Here's how the part is built. I have some questions about the finished solid (model axes, mm). Give positions to 0.01 mm unless a question says otherwise; leave off trailing zeros. Loops run counter-clockwise (first coordinate to the right, second up) from the corner with the lowest first, then second, coordinate; pieces in that order, holes last. Notation, with made-up numbers: (-39, 25) -> (-9, 25) arc R28 cw to (-9, 48) -> close; hole circle Ø10 at (88.5, -4). An arc over 180 degrees is marked (long way). Answer in a Markdown table with one row per item. Add a question column.
Item 1: If we section it at C-C (z = 13): Write out the boundary of the cut face in (x, y), then the cut area to 3 significant figures.
Item 2: If we section it at D-D (y = 132.5): Write out the boundary of the cut face in (x, z), then the cut area to 3 significant figures.
Item 3: If we section it at B-B (x = 10): Give the number of separate pieces and of enclosed holes in the cut face, then the cut area to 3 significant figures.
Item 4: If I drill on line 1 (Y direction, x = 6, z = 18); line 2 (Z direction, x = 1.75, y = 152); line 3 (Z direction, x = 7.25, y = 154), over which ranges is the centre line in solid material (lowest first)?
Item 5: If we section it at A-A (z = 18.75): Write out the boundary of the cut face in (x, y).
Item 6: We'd pull the mould along Y, two halves only. Please class faces 1 (the face through (10.14, 152.857, 4.608)), 2 (the face through (10, 151, 30)), 3 (the face through (10, 176.376, 14)), 4 (the face through (10.14, 127.33, 29.095)): released by +Y, released by -Y, zero draft, split by the parting line, or undercut.
Autodesk Inventor part; units mm, degrees
ref_plane "YZ Plane" through (0, 0, 0) normal (1, 0, 0) x (0, 1, 0)
ref_plane "XZ Plane" through (0, 0, 0) normal (0, 1, 0) x (-1, 0, 0)
ref_plane "XY Plane" through (0, 0, 0) normal (0, 0, 1) x (1, 0, 0)
sketch "Sketch1" plane through (0, 0, 0) normal (1, 0, 0) x (0, 1, 0)
  line L0 (176.3757, 0) -> (126.3757, 0)
  line L1 (126.3757, 0) -> (126.3757, 30)
  line L2 (126.3757, 30) -> (176.3757, 30)
  line L3 (176.3757, 30) -> (176.3757, 0)
  point P0 (0, 0)
  dimension "d0" = 30
  dimension "d1" = 50
extrude "Extrusion1" add sketch "Sketch1" along normal blind 20
fillet "Fillet1" radius 3.175 2 edges at (10, 126.3757, 30) (10, 176.3757, 30)
sketch "Sketch2" plane through (0, 129.5507, 30) normal (0, 0, 1) x (1, 0, 0)
  line L0 (0, 46.825) -> (20, 46.825) construction
  line L1 (10, 46.825) -> (10, -3.175) construction
  line L2 (0, -3.175) -> (20, -3.175) construction
  circle A0 centre (10, 41.825) radius 1.65
  circle A1 centre (10, 1.825) radius 1.65
  point P0 (0, -129.5507)
  dimension "d5" = 3.3
  dimension "d6" = 5
  dimension "d7" = 3.3
  dimension "d8" = 5
extrude "Extrusion2" cut sketch "Sketch2" against normal blind 30
sketch "Sketch3" plane through (20, 0, 0) normal (1, 0, 0) x (0, 0, -1)
  line L0 (-30, 173.2007) -> (-30, 129.5507) construction
  line L1 (-30, 151.3757) -> (12.6673, 151.3757) construction
  line L2 (-26.825, 126.3757) -> (0, 126.3757) construction
  line L3 (-13.4125, 126.3757) -> (-13.4125, 176.3636) construction
  circle A0 centre (-13.4125, 151.3696) radius 4
  point P0 (0, 0)
  dimension "d11" = 8
extrude "Extrusion3" cut sketch "Sketch3" against normal through all
sketch "Sketch4" plane through (20, 0, 0) normal (1, 0, 0) x (0, 0, -1)
  circle A0 centre (-13.4125, 151.3696) radius 12.5 construction
  circle A1 centre (-17.5297, 159.3727) radius 1.5 construction
  circle A2 centre (-13.4125, 151.3696) radius 5 construction
  circle A3 centre (-4.4231, 150.9337) radius 1.5 construction
  circle A4 centre (-18.2848, 143.8026) radius 1.5 construction
  circle A5 centre (-13.4125, 151.3696) radius 9 construction
  circle A6 centre (-4.4125, 151.3696) radius 1.5
  circle A7 centre (-17.9125, 159.1639) radius 1.5
  circle A8 centre (-17.9125, 143.5754) radius 1.5
  point P0 (0, 0)
  dimension "d16" = 360
extrude "Extrusion4" cut sketch "Sketch4" against normal through all
properties part number "Z Leadcrew Nut Holder"
Recorded:
| question | item | result |
|---|---|---|
| 1 | outline | (0, 126.38) -> (20, 126.38) -> (20, 147.39) -> (0, 147.39) -> close; (0, 155.35) -> (20, 155.35) -> (20, 176.38) -> (0, 176.38) -> close; hole circle Ø3.3 at (10, 131.38); hole circle Ø3.3 at (10, 171.38) |
| 1 | area | 824 mm^2 |
| 2 | outline | (0, 0) -> (8.79, 0) -> (8.79, 30) -> (0, 30) -> close; (11.21, 0) -> (20, 0) -> (20, 30) -> (11.21, 30) -> close |
| 2 | area | 528 mm^2 |
| 3 | separate pieces | 3 |
| 3 | enclosed holes | 4 |
| 3 | area | 1,230 mm^2 |
| 4 | line 1 | y = 126.38 to 142.08, 145.07 to 157.67, 160.66 to 176.38 |
| 4 | line 2 | z = 0 to 3.05, 5.77 to 9.46, 17.36 to 30 |
| 4 | line 3 | z = 0 to 10.4, 16.43 to 30 |
| 5 | outline | (0, 126.38) -> (20, 126.38) -> (20, 142.33) -> (0, 142.33) -> close; (0, 144.82) -> (20, 144.82) -> (20, 157.92) -> (0, 157.92) -> close; (0, 160.41) -> (20, 160.41) -> (20, 176.38) -> (0, 176.38) -> close; hole circle Ø3.3 at (10, 131.38); hole circle Ø3.3 at (10, 171.38) |
| 6 | face 1 | undercut |
| 6 | face 2 | zero draft |
| 6 | face 3 | released by +Y |
| 6 | face 4 | released by -Y |
